```python
from build123d import *

# Parameters (mm, degrees)
F0_R     = 1.4224
F1_DEPTH = 14.2875
F2_R     = 2.7051
F3_DEPTH = 1.4986
F4_R     = 1.27
F6_DEPTH = 0.89154


with BuildPart() as f1:
    # F0 (on Top) → F1 (new body)
    with BuildSketch(Plane.XY):
        Circle(F0_R)
    extrude(amount=F1_DEPTH)

    # F2 (on face) → F3 (join)
    with BuildSketch(Plane.XY.offset(14.2875)):
        Circle(F2_R)
    extrude(amount=F3_DEPTH)

    # F4
    f4_edges = [f1.edges().sort_by_distance(p)[0] for p in [
        (-2.7051, 0, 15.7861),
    ]]
    fillet(f4_edges, radius=F4_R)

    # F5 (on face) → F6 (cut)
    with BuildSketch(Plane.XY.offset(15.7861)):
        Polygon((0.458272, -0.79375), (0.916544, 0), (0.458272, 0.79375), (-0.458272, 0.79375), (-0.916544, 0), (-0.458272, -0.79375), align=None)
    extrude(amount=-F6_DEPTH, mode=Mode.SUBTRACT)


solid = f1.part
```
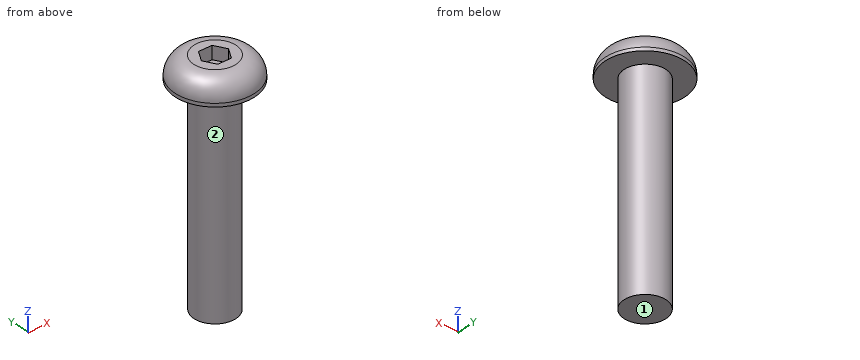
Build history of the part. All positions in model axes, mm. Face numbers are marked on the shaded views. A direction names the side the tool comes from. Give positions to 0.01 mm unless a question says otherwise; leave off trailing zeros. Order: outer loops, then holes, each group sorted by start corner. A loop starts at its lowest first (then second) coordinate and runs counter-clockwise, first axis right, second up. Notation, with made-up numbers: M 1,-11 L 52,-11 A18 ccw 52,6 Z; hole C 20.25,60 d7. An arc over 180 degrees is marked long. Return JSON: item names as keys, results as strings.
Q1. Band-saw the part on A-A (x = 0). Give the cut face in (y, z), then the cut area to 3 significant figures.
Answer list:
{"outline": "M -2.71,14.29 L -1.42,14.29 L -1.42,0 L 1.42,0 L 1.42,14.29 L 2.71,14.29 L 2.71,14.52 A1.27 ccw 1.44,15.79 L 0.79,15.79 L 0.79,14.89 L -0.79,14.89 L -0.79,15.79 L -1.44,15.79 A1.27 ccw -2.71,14.52 Z", "area": "46.6 mm^2"}
Q2. Flat gauge pins, fed straight in: pin 1 (1 mm diameter, centred on x = -1, z = 12, fed in from +Y); pin 2 (1.5 mm diameter, centred on x = -1, z = 13, fed in from -Y); pin 3 (1 mm diameter, centred on x = 2, y = 2, fed in from +Z). Where does each tip first touch, or does it go through?
Answer list:
{"pin 1": "stops at y = 1.33", "pin 2": "stops at y = -1.4", "pin 3": "stops at z = 15.42"}
Q3. 3-axis set-ups, long thin cutter, end or side, ignore diameter. For the marked faces 1 and 2: which of +Z, -Z, +X, -X, +Y, -Y reach the whole face in a straight line?
Answer list:
{"face 1": "-Z, +X, -X, +Y, -Y", "face 2": "-Z"}
Q4. Wall check: probe 1 along Z at (x, y) = (1.5, 0.35); probe 2 along Z at (x, y) = (0.4, 0.45); probe 3 along Y at (x, z) = (-1, 4.75). Give the ranges that are in metal, low to high. Write a range as from..to.
Answer list:
{"probe 1": "z = 14.29..15.78", "probe 2": "z = 0..14.89", "probe 3": "y = -1.01..1.01"}
Q5. Band-saw the part on B-B (z = 6). Give the cut face in (x, y).
Answer list:
{"outline": "C 0,0 d2.84"}
